Design review of the part built by this model. Coordinates are the model's own, in mm. Round coordinates to 2 decimals unless told otherwise and drop trailing zeros. Order: outer loops, then holes, each group sorted by start corner. A loop starts at its lowest first (then second) coordinate and runs counter-clockwise, first axis right, second up.
from build123d import *

# Parameters (mm, degrees)
F0_W     = 3.977105
F0_H     = 5.380789
F0_W_2   = 4.678948
F0_H_2   = 3.041315
F0_W_3   = 5.146842
F0_H_3   = 6.31658
F0_H_4   = 5.380787
F0_H_5   = 8.188158
F0_W_4   = 3.509209
F0_W_5   = 4.444998
F0_R     = 4.004533
F1_DEPTH = 2.54


with BuildPart() as f1:
    # F0 (on Front) → F1 (new body)
    with BuildSketch(Plane.XZ):
        Polygon((19.885525, -32.050792), (19.885525, 35.326052), (-22.926843, 36.027897), (-22.926843, -31.348947), align=None)
        with Locations((-18.364869, 6.901447)):
            Rectangle(F0_W, F0_H, mode=Mode.SUBTRACT)
        with Locations((-10.761579, 5.731711)):
            Rectangle(F0_W_2, F0_H_2, mode=Mode.SUBTRACT)
        with Locations((-2.573421, 6.901447)):
            Rectangle(F0_W_3, F0_H, mode=Mode.SUBTRACT)
        with Locations((-18.364869, 19.300658)):
            Rectangle(F0_W, F0_H_3, mode=Mode.SUBTRACT)
        with Locations((-18.364869, 30.062235)):
            Rectangle(F0_W, F0_H_4, mode=Mode.SUBTRACT)
        with Locations((-10.761579, 19.300658)):
            Rectangle(F0_W_2, F0_H_3, mode=Mode.SUBTRACT)
        with Locations((-2.573421, 18.364869)):
            Rectangle(F0_W_3, F0_H_5, mode=Mode.SUBTRACT)
        Polygon((-13.568947, 27.371842), (-13.101053, 32.752629), (-8.422105, 32.752629), (-8.422105, 27.371842), align=None, mode=Mode.SUBTRACT)
        Polygon((-5.38079, 27.371842), (-5.146842, 32.752629), (0, 32.752629), (0, 27.371842), align=None, mode=Mode.SUBTRACT)
        with Locations((5.965658, 6.901447)):
            Rectangle(F0_W_4, F0_H, mode=Mode.SUBTRACT)
        with Locations((5.965658, 19.300658)):
            Rectangle(F0_W_4, F0_H_3, mode=Mode.SUBTRACT)
        Polygon((3.275263, 27.371842), (4.211054, 32.752629), (7.720263, 32.752629), (7.720263, 27.371842), align=None, mode=Mode.SUBTRACT)
        with Locations((14.153816, 19.300658)):
            Rectangle(F0_W_5, F0_H_3, mode=Mode.SUBTRACT)
        Polygon((10.995527, 27.371842), (11.931317, 32.752629), (16.376315, 32.752629), (16.376315, 27.371842), align=None, mode=Mode.SUBTRACT)
        Polygon((19.885525, -43.514211), (19.885525, -32.050792), (-22.926843, -31.348947), (-22.926843, -43.514211), align=None)
        with Locations((0, -37.665527)):
            Circle(F0_R, mode=Mode.SUBTRACT)
        with Locations((0, -37.665527)):
            Circle(F0_R)
    extrude(amount=F1_DEPTH)


solid = f1.part
1) To check wall thickness, follow line 1 along X through (y, z) = (-1, 19); line 2 along Z through (x, y) = (-4.5, -1.05); line 3 along Z through (x, y) = (14, -1.5). State the ranges of each line that lie inside material, in increasing order.
Results:
line 1: x = -22.93 to -20.35, -16.38 to -13.1, -8.42 to -5.15, 0 to 4.21, 7.72 to 11.93, 16.38 to 19.89
line 2: z = -43.51 to 4.21, 9.59 to 14.27, 22.46 to 27.37, 32.75 to 35.73
line 3: z = -43.51 to 16.14, 22.46 to 27.37, 32.75 to 35.42
2) The part is to be moulded in two halves that separate along Z. For faces 1 (the face through (-2, -1, -43.514)), 2 (the face through (-13.101, -1, 6)), say which applies: released by +Z, released by -Z, zero draft, split by the parting line, or undercut.
Results:
face 1: released by -Z
face 2: undercut
3) Take a section at B-B on x = -18. Give the boundary of the cut face in (y, z), plus the area to 3 significant figures.
Results:
outline: (-2.54, -43.51) - (0, -43.51) - (0, 4.21) - (-2.54, 4.21) - close; (-2.54, 9.59) - (0, 9.59) - (0, 16.14) - (-2.54, 16.14) - close; (-2.54, 22.46) - (0, 22.46) - (0, 27.37) - (-2.54, 27.37) - close; (-2.54, 32.75) - (0, 32.75) - (0, 35.95) - (-2.54, 35.95) - close
area: 158 mm2
4) Take a section at A-A on z = 15. Give the boundary of the cut face in (x, y), plus the area to 3 significant figures.
Results:
outline: (-22.93, -2.54) - (-5.15, -2.54) - (-5.15, 0) - (-22.93, 0) - close; (0, -2.54) - (19.89, -2.54) - (19.89, 0) - (0, 0) - close
area: 95.7 mm2
5) Take a section at C-C on z = 6.5. Give the boundary of the cut face in (x, y).
Results:
outline: (-22.93, -2.54) - (-20.35, -2.54) - (-20.35, 0) - (-22.93, 0) - close; (-16.38, -2.54) - (-13.1, -2.54) - (-13.1, 0) - (-16.38, 0) - close; (-8.42, -2.54) - (-5.15, -2.54) - (-5.15, 0) - (-8.42, 0) - close; (0, -2.54) - (4.21, -2.54) - (4.21, 0) - (0, 0) - close; (7.72, -2.54) - (19.89, -2.54) - (19.89, 0) - (7.72, 0) - close
6) Clearance check with a flat-ended pin moving along its axis: P1, Ø1.3, axis at x = 5, y = -1, coming from the +Z side. State where the tip first meets the part, or that it passes through.
Results:
P1: stops at z = 35.58
7) Take a section at D-D on x = 15. Give the boundary of the cut face in (y, z).
Results:
outline: (-2.54, -43.51) - (0, -43.51) - (0, 16.14) - (-2.54, 16.14) - close; (-2.54, 22.46) - (0, 22.46) - (0, 27.37) - (-2.54, 27.37) - close; (-2.54, 32.75) - (0, 32.75) - (0, 35.41) - (-2.54, 35.41) - close
